Study the drawing (mm; zero at the part's minimum x, y, z) and answer. Round coordinates to 2 decimals unless told otherwise and drop trailing zeros. Order: outer loops, then holes, each group sorted by start corner. A loop starts at its lowest first (then second) coordinate and runs counter-clockwise, first axis right, second up. Notation, with made-up numbers: M 13,-8.5 L 39,-8.5 A28 cw 39,17.5 Z; hole C 51.5,81.25 d7. An arc over 180 degrees is marked long. Put each result on its own line as item: value. Start each with the question number.
1. Each of these flat-tipped pins is pushed along its axis until it touches: pin 1 Ø1.7 at (y, z) = (30.5, 205) entering from -X; pin 2 Ø1 at (x, z) = (39, 128) entering from -Y; pin 3 Ø12 at (x, z) = (25, 56.5) entering from +Y; pin 4 Ø4 at (x, y) = (33.5, 32.5) entering from +Z (1 decimal). Where does it stop, or does it pass through?
2. The part is cut by section A-A (y = 31.75). Give the vertices of the cut face in (x, z).
3. Consider line 1 (Y direction, x = 30.5, z = 77.5) (1 decimal); line 2 (X direction, y = 32.5, z = 136); line 3 (Z direction, x = 31, y = 51). Determine where each line is inside the solid, lowest interval first.
4. The part is cut by section B-B (z = 28). Give the vertices of the cut face in (x, y).
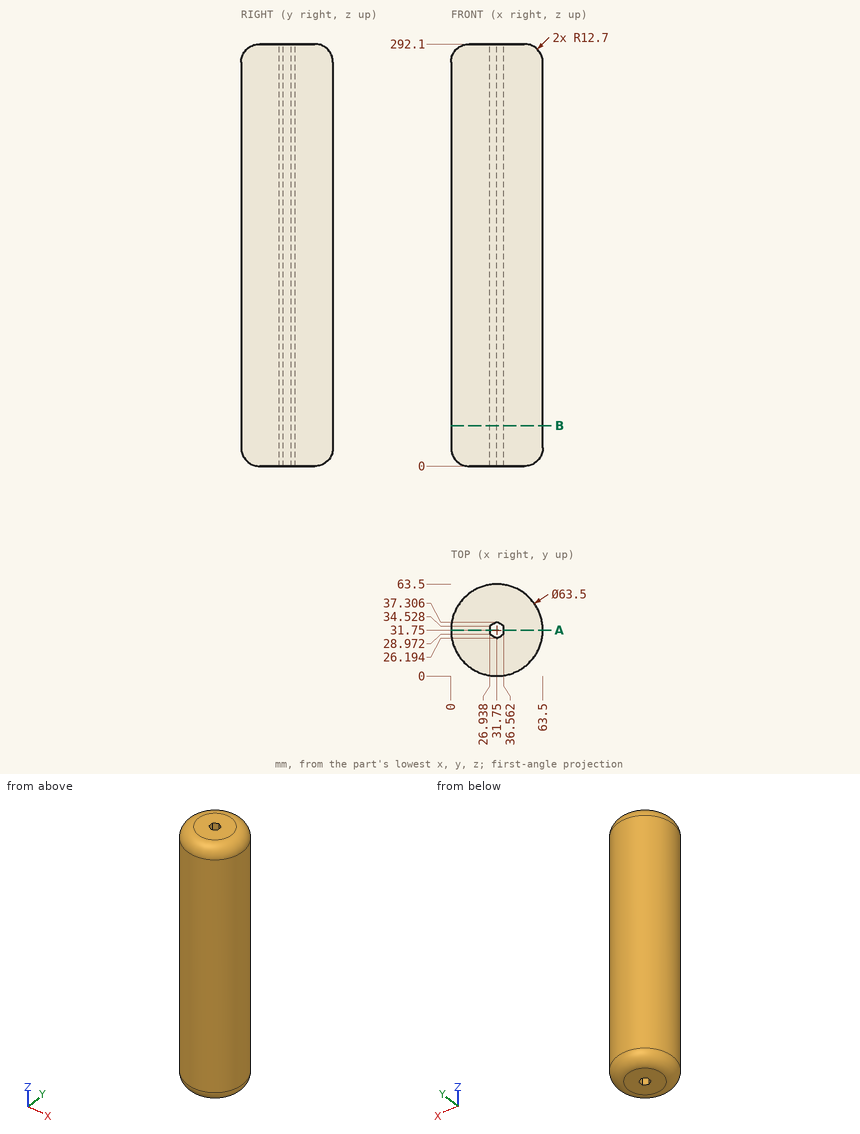
Resolved:
1. pin 1: x = 0
1. pin 2: y = 0.73
1. pin 3: y = 63.49
1. pin 4: through
2. outline: M 0,12.7 A12.7 ccw 12.7,0 L 26.94,0 L 26.94,292.1 L 12.7,292.1 A12.7 ccw 0,279.4 Z; M 36.56,0 L 50.8,0 A12.7 ccw 63.5,12.7 L 63.5,279.4 A12.7 ccw 50.8,292.1 L 36.56,292.1 Z
3. line 1: 0 to 26.9, 36.6 to 63.5
3. line 2: 0.01 to 26.94, 36.56 to 63.49
3. line 3: 0 to 292.1
4. outline: C 31.75,31.75 d63.5; hole M 26.94,28.97 L 31.75,26.19 L 36.56,28.97 L 36.56,34.53 L 31.75,37.31 L 26.94,34.53 Z
